Can you work these out from the model? Positions are in its coordinate system, mm. Face numbers are marked on the shaded views. A direction names the side the tool comes from. Give positions to 0.01 mm unless a question says otherwise; leave off trailing zeros. Order: outer loops, then holes, each group sorted by start corner. A loop starts at its lowest first (then second) coordinate and runs counter-clockwise, first axis right, second up. Notation, with made-up numbers: M -20,36.5 L 26,36.5 A22 ccw 26,59.5 Z; hole C 9.5,84 d3. An arc over 180 degrees is marked long. Use a Markdown table: item, result. Add a question column.
from build123d import *

# Parameters (mm, degrees)
F0_W    = 50
F0_H    = 50
F2_W    = 33.4539487958
F2_H    = 22.2039483488
F5_SIZE = 10


# Not quite as in the source:
# - a fillet or chamfer that OpenCascade refuses, or shapes differently, is made with other operations: its cross-section is extruded or revolved along the edge and cut away or added


with BuildPart() as f1:
    # F0 (on Front) → F1 (revolve)
    with BuildSketch(Plane.XZ):
        with Locations((-25, 25)):
            Rectangle(F0_W, F0_H)
    revolve(axis=Axis((0, 0, 25), (0, 0, 1)))

    # F2 (on Front) → F3 (revolve)
    with BuildSketch(Plane.XZ):
        with Locations((-16.7269743979, 46.6282907873)):
            Rectangle(F2_W, F2_H)
    revolve(axis=Axis((0, 0, 50), (0, 0, -1)))

    # F4: fillet of radius 61.079603128 on 1 edges, made by hand

    # F4_s1 → F4_t2 (revolve, cut)
    with BuildSketch(Plane.XZ):
        with BuildLine():
            ThreePointArc((-33.4539487958, 50), (-19.0772136264, 55.7661180216), (-3.7122939075, 57.7302649617))
            Line((-3.7122939075, 57.7302649617), (-33.4539487958, 57.7302649617))
            Line((-33.4539487958, 57.7302649617), (-33.4539487958, 50))
        make_face()
    revolve(axis=Axis((0, 0, 57.7302649617), (0, 0, -1)), mode=Mode.SUBTRACT)

    # F5
    f5_edges = [f1.edges().sort_by_distance(p)[0] for p in [
        (50, 0, 50),
    ]]
    chamfer(f5_edges, length=F5_SIZE)


solid = f1.part
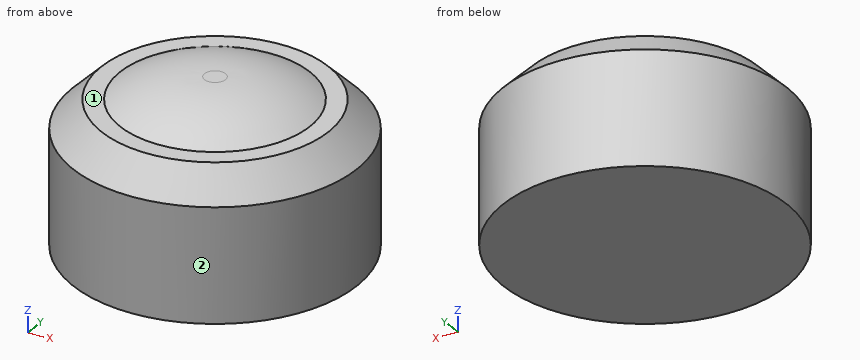
1. On a 3-axis mill with a long thin cutter (end or side, diameter ignored), from which of +Z, -Z, +X, -X, +Y, -Y can I reach the whole of each face in a straight line? I mean the marked faces 1 and 2. Say none if no direction works.
2. I need wall thicknesses on L1, parallel to Z at x = -18.5, y = -34; L2, parallel to X at y = 0.5, z = 28.5; L3, parallel to Y at x = -11, z = 45. Which ranges of each line are inside material? Lowest first, please. Write a range as [from, to].
3. If we section it at A-A, the plane z = 13: List the corners of the cut face in (x, y) for me, then the cut area to 3 significant figures.
4. Will these pins go through, and if not, where does the flat tip stop? pin 1 (1 mm diameter, centred on y = -23.5, z = 40.5, fed in from -X); pin 2 (1.5 mm diameter, centred on y = -11.5, z = 49.5, fed in from +X); pin 3 (12 mm diameter, centred on y = -36, z = 40, fed in from -X).
Geometry results:
| question | item | result |
|---|---|---|
| 1 | face 1 | +Z |
| 1 | face 2 | +Z, -Z |
| 2 | L1 | z = [0, 50] |
| 2 | L2 | x = [-50, 50] |
| 2 | L3 | y = [-43.63, 43.63] |
| 3 | outline | C 0,0 d100 |
| 3 | area | 7,850 mm^2 |
| 4 | pin 1 | stops at x = -44.19 |
| 4 | pin 2 | stops at x = 39.64 |
| 4 | pin 3 | stops at x = -40 |
